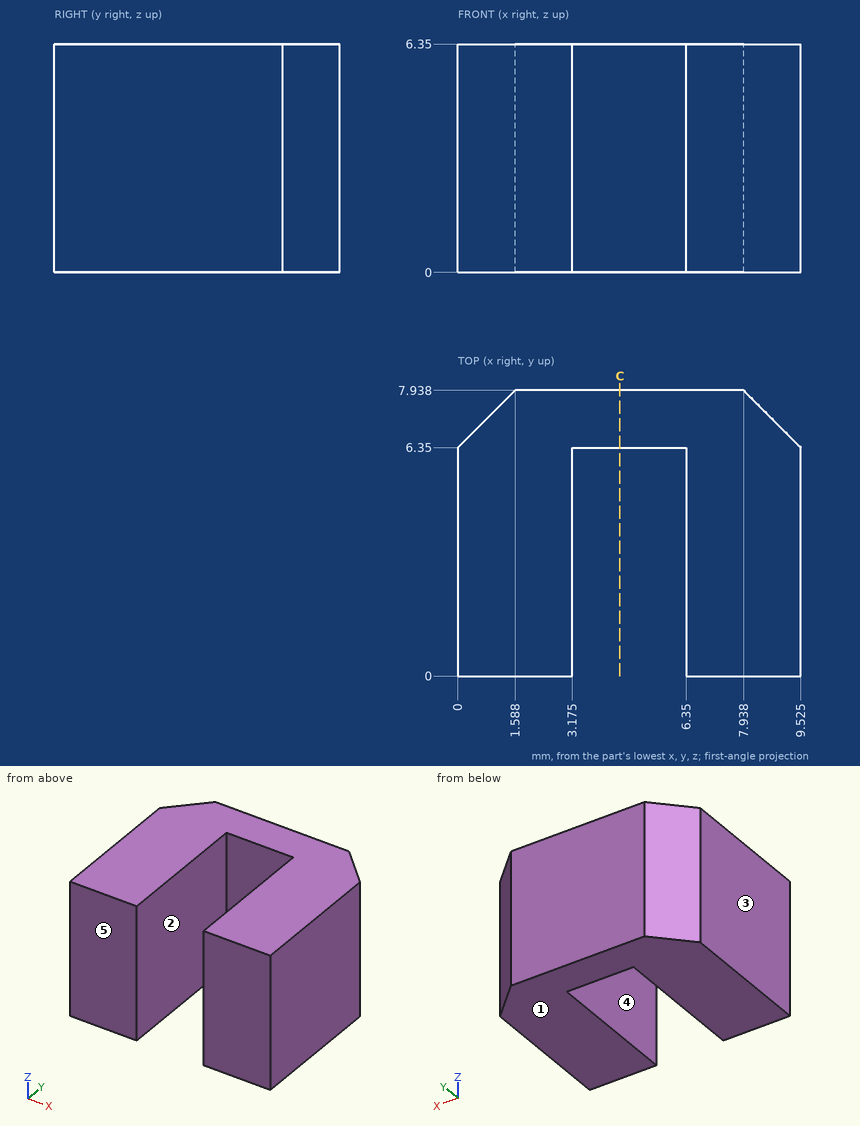
Source: three-view drawing plus pictorial views. Frame: mm from the lowest corner of the part. A direction names the side the tool comes from. Round coordinates to 2 decimals unless told otherwise and drop trailing zeros. Write each loop counter-clockwise with the first axis right and the second up, starting at its lowest first coordinate (ties: lowest second). Pieces come first, ordered by that corner, then holes. Notation, with made-up numbers: M 66,58 L 120,58 A15 cw 120,78 Z; hole C 59.25,-39 d3. An arc over 180 degrees is marked long. Write item = value, one per line.
Item 1: Access query for the marked faces 4 and 5. Directions: +Z, -Z, +X, -X, +Y, -Y. A direction counts if a zero-diameter tool reaches every point of the face in a straight line with its end or side. Return the directions, or none.
Findings:
face_4 = +Z, -Z, -Y
face_5 = +Z, -Z, +X, -X, -Y
Item 2: Material intervals for line 1 along Y through (x, z) = (6, 1.25); line 2 along Y through (x, z) = (9, 1.75) (1 decimal); line 3 along X through (y, z) = (6.75, 5) (1 decimal), sorted ascending. Write a range as [from, to].
Findings:
line_1 = [6.35, 7.94]
line_2 = [0, 6.9]
line_3 = [0.4, 9.1]
Item 3: Pull-direction query (X, two-part tool) for the marked faces 1, 2 and 3; classes: pulls with the +X half, pulls with the -X half, needs draft (parallel to the pull), parting line crosses it, or undercut.
Findings:
face_1 = needs draft
face_2 = undercut
face_3 = pulls with the -X half
Item 4: Pin query (flat end, axial travel): P1, Ø2.5, axis at x = 5, z = 3.5, coming from the -Y side; P2, Ø3, axis at x = 8, z = 4.5, coming from the -Y side. Return the tip coordinate at first contact, or that it passes through.
Findings:
P1 = 6.35
P2 = 0
Item 5: Section query C-C on x = 4.5. Return loops of the section in (y, z).
Findings:
outline = M 6.35,0 L 7.94,0 L 7.94,6.35 L 6.35,6.35 Z
